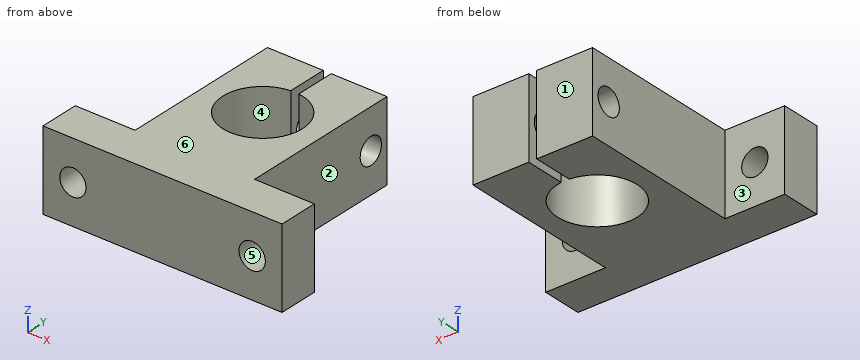
```python
from build123d import *

# Parameters (mm, degrees)
BOSS_EXTRUDE1_DEPTH = 10
SKETCH3_R           = 10
CUT_EXTRUDE1_DEPTH  = 26
SKETCH9_R           = 3.3
CUT_EXTRUDE2_DEPTH  = 26
SKETCH10_R          = 3.3
CUT_EXTRUDE3_DEPTH  = 26
SKETCH12_R          = 3.3
CUT_EXTRUDE5_DEPTH  = 46
SKETCH15_W          = 2
SKETCH15_H          = 20
CUT_EXTRUDE7_DEPTH  = 15


with BuildPart() as part:
    # Sketch2 → Boss-Extrude1 (new, symmetric)
    with BuildSketch(Plane.XY):
        Polygon((45, 10), (60, 10), (60, 0), (0, 0), (0, 10), (15, 10), (15, 51), (45, 51), align=None)
    extrude(amount=BOSS_EXTRUDE1_DEPTH, both=True)

    # Sketch3 → Cut-Extrude1 (cut)
    with BuildSketch(Plane.XY.offset(10)):
        with Locations((30, 31)):
            Circle(SKETCH3_R)
    extrude(amount=-CUT_EXTRUDE1_DEPTH, mode=Mode.SUBTRACT)

    # Sketch9 → Cut-Extrude2 (cut)
    with BuildSketch(Plane(origin=(0, 10, 0), x_dir=(1, 0, 0), z_dir=(0, 1, 0))):
        with Locations(Location((7.5, 0, 0), (0, 0, 270))):
            Circle(SKETCH9_R)
    extrude(amount=-CUT_EXTRUDE2_DEPTH, mode=Mode.SUBTRACT)

    # Sketch10 → Cut-Extrude3 (cut)
    with BuildSketch(Plane(origin=(0, 10, 0), x_dir=(1, 0, 0), z_dir=(0, 1, 0))):
        with Locations(Location((52.5, 0, 0), (0, 0, 270))):
            Circle(SKETCH10_R)
    extrude(amount=-CUT_EXTRUDE3_DEPTH, mode=Mode.SUBTRACT)

    # Sketch12 → Cut-Extrude5 (cut)
    with BuildSketch(Plane.ZY.offset(-15)):
        with Locations((0, 46)):
            Circle(SKETCH12_R)
    extrude(amount=-CUT_EXTRUDE5_DEPTH, mode=Mode.SUBTRACT)

    # Sketch15 → Cut-Extrude7 (cut)
    with BuildSketch(Plane(origin=(0, 51, 0), x_dir=(1, 0, 0), z_dir=(0, 1, 0))):
        with Locations((30, 0)):
            Rectangle(SKETCH15_W, SKETCH15_H)
    extrude(amount=-CUT_EXTRUDE7_DEPTH, mode=Mode.SUBTRACT)


solid = part.part
```
Part model, mm, in its own coordinate system. Face numbers are marked on the shaded views. A direction names the side the tool comes from. Round coordinates to 2 decimals unless told otherwise and drop trailing zeros. Loops run counter-clockwise (first coordinate to the right, second up) from the corner with the lowest first, then second, coordinate; pieces in that order, holes last.
1. Slice it at D-D (x = 42.5). Give the cut face in (y, z), and give its area (3 significant figures).
Solutions:
outline: (0, -10) - (51, -10) - (51, 10) - (0, 10) - close; hole circle Ø6.6 at (46, 0)
area: 986 mm2
2. Slice it at C-C (z = 8.5). Give the cut face in (x, y).
Solutions:
outline: (0, 0) - (60, 0) - (60, 10) - (45, 10) - (45, 51) - (31, 51) - (31, 40.95) arc R10 cw (long way) to (29, 40.95) - (29, 51) - (15, 51) - (15, 10) - (0, 10) - close
3. Flat gauge pins, fed straight in: pin 1 (10 mm diameter, centred on y = 33.5, z = 0, fed in from +X); pin 2 (3 mm diameter, centred on y = 36.5, z = 4, fed in from -X). Where does each tip first touch, or does it go through?
Solutions:
pin 1: stops at x = 45
pin 2: stops at x = 15
4. 3-axis set-ups, long thin cutter, end or side, ignore diameter. For the marked faces 1, 2 and 3: which of +Z, -Z, +X, -X, +Y, -Y reach the whole face in a straight line?
Solutions:
face 1: +Z, -Z, +X, -X, +Y
face 2: +Z, -Z, +X, +Y
face 3: +Z, -Z, -X, +Y
5. Drill centre lines: line 1 along X through (y, z) = (3.25, 0); line 2 along X through (y, z) = (43.5, -5); line 3 along X through (y, z) = (30.5, -6.5). Where is each one in solid material? Low to high.
Solutions:
line 1: x = 0 to 4.2, 10.8 to 49.2, 55.8 to 60
line 2: x = 15 to 29, 31 to 45
line 3: x = 15 to 20.01, 39.99 to 45
6. Slice it at B-B (x = 52.5). Give the cut face in (y, z), and give its area (3 significant figures).
Solutions:
outline: (0, -10) - (10, -10) - (10, -3.3) - (0, -3.3) - close; (0, 3.3) - (10, 3.3) - (10, 10) - (0, 10) - close
area: 134 mm2
7. Slice it at A-A (y = 31). Give the cut face in (x, z).
Solutions:
outline: (15, -10) - (20, -10) - (20, 10) - (15, 10) - close; (40, -10) - (45, -10) - (45, 10) - (40, 10) - close
8. Two-plate mould, pull along Z, no slides. Class the marked faces 4, 5 and 6: pulls with the +Z half, pulls with the -Z half, needs draft (parallel to the pull), parting line crosses it, or undercut.
Solutions:
face 4: needs draft
face 5: undercut
face 6: pulls with the +Z half
